from build123d import *

# Parameters (mm, degrees)
F1_DEPTH = 12.7


with BuildPart() as f1:
    # F0 (on Front) → F1 (new body, symmetric)
    with BuildSketch(Plane.XZ):
        with BuildLine():
            ThreePointArc((-54.047783, -35.329167), (18.431438, -61.883721), (64.570217, 0))
            ThreePointArc((64.570217, 0), (16.705627, 62.371748), (-55.926047, 32.273676))
            Line((-55.926047, 32.273676), (0, 32.273676))
            Line((0, 32.273676), (0, -35.329167))
            Line((0, -35.329167), (-54.047783, -35.329167))
        make_face()
    extrude(amount=F1_DEPTH, both=True)


solid = f1.part
For this review, take the finished solid that the model builds, in its own axes (mm). A direction names the side the tool comes from. Give positions to 0.01 mm unless a question says otherwise; leave off trailing zeros. Loops run counter-clockwise (first coordinate to the right, second up) from the corner with the lowest first, then second, coordinate; pieces in that order, holes last.
Item 1: Draft analysis for pull direction Z (two halves, no side actions). For faces 3 (the flat face through (0, 0, -1)), 4 (the flat face through (17, 12.7, 1)), state which applies: +Z half, -Z half, draft (parallel to the pull), parting line (faces both ways), or undercut.
Item 2: For line 1 along Z through (x, y) = (-2, -5.25); line 2 along Z through (x, y) = (-41, -3); line 3 along Z through (x, y) = (6.5, -1.75), list the stretches that pass through material, from the lowest coordinate up.
Item 3: Take a section at C-C, the plane x = 45. State the section outline as (y, z) points, and give its area (3 significant figures).
Item 4: Take a section at B-B, the plane z = -33.5. State the section outline as (x, y) points.
Item 5: Tool access review of faces 1 (the flat face through (-27, 0, -35.329)), 2 (the flat face through (17, -12.7, 1)): name each direction out of +Z, -Z, +X, -X, +Y, -Y from which nothing blocks a thin tool from reaching the whole face with its end or side.
Item 6: Take a section at A-A, the plane y = 1. State the section outline as (x, z) points.
Item 7: Insertion check: pin 1 (7.5 mm diameter, centred on x = -14, y = -1.5, fed in from +Z); pin 2 (1.5 mm diameter, centred on y = 3, z = -41, fed in from +X); pin 3 (12.5 mm diameter, centred on y = 3, z = 15, fed in from -X). Each pin has a flat end and moves straight along its axis. Give the tip position at first contact, or say it passes through.
Calculated:
1. face 3: undercut
1. face 4: draft
2. line 1: z = -64.54 to -35.33, 32.27 to 64.54
2. line 2: z = -49.88 to -35.33, 32.27 to 49.88
2. line 3: z = -64.24 to 64.24
3. outline: (-12.7, -46.31) - (12.7, -46.31) - (12.7, 46.31) - (-12.7, 46.31) - close
3. area: 2,350 mm2
4. outline: (0, -12.7) - (55.2, -12.7) - (55.2, 12.7) - (0, 12.7) - close
5. face 1: -X, +Y, -Y
5. face 2: +Z, -Z, +X, -X, -Y
6. outline: (-55.93, 32.27) - (0, 32.27) - (0, -35.33) - (-54.05, -35.33) arc R64.57 ccw (long way) to start
7. pin 1: stops at z = 63.75
7. pin 2: stops at x = 50.49
7. pin 3: stops at x = 0
